The model under review builds one solid part; all positions refer to its coordinate system, in mm. Face numbers are marked on the shaded views. A direction names the side the tool comes from. Coordinates: 2 decimals unless noted, no trailing zeros. Loops run counter-clockwise (first coordinate to the right, second up) from the corner with the lowest first, then second, coordinate; pieces in that order, holes last. Notation, with made-up numbers: M 89.25,36.25 L 127.25,36.25 A25 cw 127.25,64.25 Z; hole C 28.5,83.5 d10. An arc over 180 degrees is marked long. Use CSV: the item, a comma, the result in double quotes. Start each with the question number.
1. Add section C-C, the plane x = -1. Write out the cut boundary in (y, z), then the cut area to 3 significant figures.
2. Add section D-D, the plane y = 4. Write out the cut boundary in (x, z).
3. Tool access review of the marked faces 1, 2 and 3: name each direction out of +Z, -Z, +X, -X, +Y, -Y from which nothing blocks a thin tool from reaching the whole face with its end or side.
4. Draft analysis for pull direction X (two halves, no side actions). For the marked faces 4, 5 and 6, state which applies: +X half, -X half, draft (parallel to the pull), parting line (faces both ways), or undercut.
5. Clearance check with flat-ended pins moving along their axes: P1, Ø6, axis at x = -2.5, z = -2.5, coming from the -Y side; P2, Ø4, axis at x = -4.5, y = 0, coming from the +Z side; P3, Ø4.5, axis at x = -3, z = 3.5, coming from the +Y side; P4, Ø4, axis at x = -1, y = 4, coming from the +Z side. State where each tip first meets the part, or that it passes through.
6. Add section B-B, the plane z = 17.5. Write out the cut boundary in (x, y).
7. For L1, parallel to Z at x = 0, y = 0; L2, parallel to X at y = -2, z = 17.5; L3, parallel to Y at x = 3, z = 4.5, list the stretches that pass through material, from the lowest coordinate up.
8. Add section A-A, the plane y = 1.75. Write out the cut boundary in (x, z).
from build123d import *

# Parameters (mm, degrees)
F1_DEPTH = 7.5
F2_DEPTH = 3.45
F4_D     = 4


with BuildPart() as f1:
    # F0 (on Front) → F1 (new body, symmetric)
    with BuildSketch(Plane.XZ):
        with BuildLine():
            Line((-7.5, 34), (-7.5, 1.74356))
            ThreePointArc((-7.5, 1.74356), (-4.788768, 6.029735), (0, 7.7))
            ThreePointArc((0, 7.7), (4.787697, 6.030585), (7.49938, 1.746224))
            Line((7.49938, 1.746224), (7.49938, 29.096422))
            ThreePointArc((7.49938, 29.096422), (7.206487, 29.803529), (6.49938, 30.096422))
            ThreePointArc((6.49938, 30.096422), (4.696258, 29.349544), (3.94938, 27.546422))
            Line((3.94938, 27.546422), (3.95, 12.5))
            ThreePointArc((3.95, 12.5), (0, 8.55), (-3.95, 12.5))
            Line((-3.95, 12.5), (-3.95, 32.45))
            ThreePointArc((-3.95, 32.45), (-4.696878, 34.253122), (-6.5, 35))
            ThreePointArc((-6.5, 35), (-7.207107, 34.707107), (-7.5, 34))
        make_face()
    extrude(amount=F1_DEPTH, both=True)

    # F0 (on Front) → F2 (join, symmetric)
    with BuildSketch(Plane.XZ):
        with BuildLine():
            Line((0, 0), (-7.5, 0))
            ThreePointArc((-7.5, 0), (-0.00031, -7.49969), (7.49938, 0))
            Line((7.49938, 0), (0, 0))
        make_face()
        with BuildLine():
            Line((-7.5, 1.74356), (-7.5, 0))
            Line((-7.5, 0), (0, 0))
            Line((0, 0), (0, 7.7))
            ThreePointArc((0, 7.7), (-4.788768, 6.029735), (-7.5, 1.74356))
        make_face()
        with BuildLine():
            Line((0, 0), (7.49938, 0))
            Line((7.49938, 0), (7.49938, 1.746224))
            ThreePointArc((7.49938, 1.746224), (4.787697, 6.030585), (0, 7.7))
            Line((0, 7.7), (0, 0))
        make_face()
    extrude(amount=F2_DEPTH, both=True)

    # F4 (through all)
    with Locations(Plane.XZ.offset(3.45)):
        with Locations((0, 0)):
            Hole(F4_D / 2)


solid = f1.part
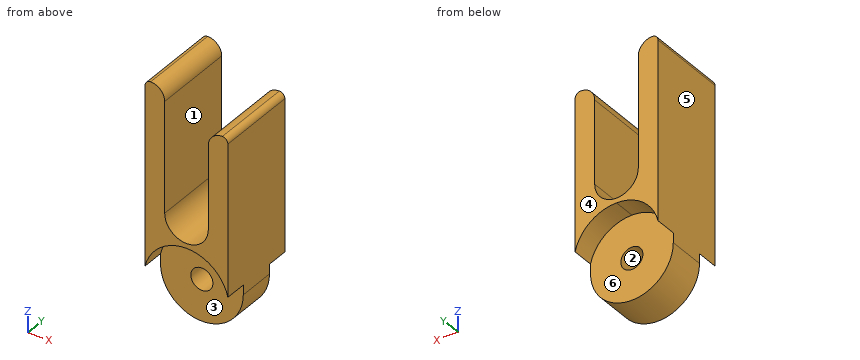
Computed:
1,outline,"M -7.5,7.63 L -3.45,7.63 L -3.45,1.73 L 3.45,1.73 L 3.45,7.63 L 7.5,7.63 L 7.5,8.68 L -7.5,8.68 Z; M -3.45,-7.43 L 3.45,-7.43 L 3.45,-1.73 L -3.45,-1.73 Z"
1,area,"95.7 mm^2"
2,outline,"M -7.5,1.74 A7.7 cw 7.5,1.75 L 7.5,29.1 A1 ccw 6.5,30.1 A2.55 ccw 3.95,27.55 L 3.95,12.5 A3.95 cw -3.95,12.5 L -3.95,32.45 A2.55 ccw -6.5,35 A1 ccw -7.5,34 Z"
3,face 1,"+Z, +Y, -Y"
3,face 2,"+Y, -Y"
3,face 3,"-Z, -Y"
4,face 4,"draft"
4,face 5,"-X half"
4,face 6,"undercut"
5,P1,"stops at y = -3.45"
5,P2,"stops at z = 35"
5,P3,"stops at y = 3.45"
5,P4,"stops at z = 9.93"
6,outline,"M -7.5,-7.5 L -3.95,-7.5 L -3.95,7.5 L -7.5,7.5 Z; M 3.95,-7.5 L 7.5,-7.5 L 7.5,7.5 L 3.95,7.5 Z"
7,L1,"z = -7.5 to -2, 2 to 8.55"
7,L2,"x = -7.5 to -3.95, 3.95 to 7.5"
7,L3,"y = -3.45 to 3.45"
8,outline,"M -7.5,0 A7.5 ccw 7.5,0 L 7.5,29.1 A1 ccw 6.5,30.1 A2.55 ccw 3.95,27.55 L 3.95,12.5 A3.95 cw -3.95,12.5 L -3.95,32.45 A2.55 ccw -6.5,35 A1 ccw -7.5,34 Z; hole C 0,0 d4"
